Can you work these out from the model? Positions are in its coordinate system, mm. Give positions to 0.01 mm unless a question says otherwise; leave off trailing zeros. Loops run counter-clockwise (first coordinate to the right, second up) from the corner with the lowest first, then second, coordinate; pieces in that order, holes last. Notation, with made-up numbers: M 35,-23.75 L 87,-23.75 A34 cw 87,6.25 Z; hole C 54.5,-29 d6. An arc over 180 degrees is marked long. Put each result on its own line as item: value. Start each with the question number.
1) Imagine slicing it at D-D (z = 64.5). Write out the boundary of the cut face in (x, y), then the cut area to 3 significant figures.
2) Please list where these lines run through material, in increasing order: line 1 along Y through (x, z) = (0, 303.25); line 2 along Z through (x, y) = (3.5, -1.5); line 3 along Z through (x, y) = (4.25, 5). Write a range as from..to.
3) Imagine slicing it at A-A (y = 0). Write out the boundary of the cut face in (x, z).
4) Imagine slicing it at C-C (z = 30). Write out the boundary of the cut face in (x, y).
5) For P1, Ø3, axis at x = -5.5, z = 180.5, coming from the +Y side; P2, Ø8, axis at x = 0, y = 0, coming from the +Z side; P3, Ø1, axis at y = -2.5, z = 168, coming from the +X side, each with a flat end and sliding along its axis, tell me the tip position at first contact or that it passes through.
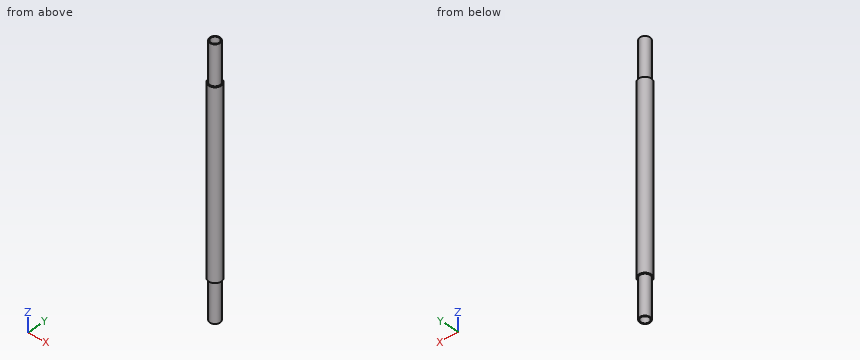
Autodesk Inventor part; units mm, degrees
ref_plane "YZ Plane" through (0, 0, 0) normal (1, 0, 0) x (0, 1, 0)
ref_plane "XZ Plane" through (0, 0, 0) normal (0, 1, 0) x (-1, 0, 0)
ref_plane "XY Plane" through (0, 0, 0) normal (0, 0, 1) x (1, 0, 0)
sketch "Sketch1" plane through (0, 0, 0) normal (0, 0, 1) x (1, 0, 0)
  circle A0 centre (0, 0) radius 7.5
  dimension "d0" = 15
extrude "Extrusion1" add sketch "Sketch1" along normal blind 307
sketch "Sketch2" plane through (0, 0, 307) normal (0, 0, 1) x (1, 0, 0)
  circle A0 centre (0, 0) radius 6
  circle A1 centre (0, 0) radius 7.5
  dimension "d3" = 12
extrude "Extrusion2" cut sketch "Sketch2" against normal blind 46
sketch "Sketch3" plane through (0, 0, 307) normal (0, 0, 1) x (1, 0, 0)
  circle A0 centre (0, 0) radius 5
  dimension "d6" = 10
extrude "Extrusion3" cut sketch "Sketch3" against normal blind 12
sketch "Sketch4" plane through (0, 0, 0) normal (0, 0, -1) x (-1, 0, 0)
  circle A0 centre (0, 0) radius 5
  circle A1 centre (0, 0) radius 7.5
  circle A2 centre (0, 0) radius 6
  circle A3 centre (0, 0) radius 5
  dimension "d9" = 15
extrude "Extrusion4" cut sketch "Sketch4" against normal blind 46 contours A1
sketch "Sketch5" plane through (0, 0, 0) normal (0, 0, -1) x (-1, 0, 0)
  circle A0 centre (0, 0) radius 5
  dimension "d12" = 10
extrude "Extrusion5" cut sketch "Sketch5" against normal blind 12
Recorded:
1. outline: C 0,0 d15
1. area: 177 mm²
2. line 1: -6..-5, 5..6
2. line 2: 12..295
2. line 3: 46..261
3. outline: M -7.5,46 L -6,46 L -6,0 L -5,0 L -5,12 L 5,12 L 5,0 L 6,0 L 6,46 L 7.5,46 L 7.5,261 L 6,261 L 6,307 L 5,307 L 5,295 L -5,295 L -5,307 L -6,307 L -6,261 L -7.5,261 Z
4. outline: C 0,0 d12
5. P1: y = 6.34
5. P2: z = 295
5. P3: x = 7.23
